```python
from build123d import *

# Parameters (mm, degrees)
DODANIE_WYCI_GNI_CIE1_DEPTH                 = 880
DODANIE_WYCI_GNI_CIE1_DEPTH_BACK            = 880
SZKIC1_R                                    = 12
WYTNIJ_WYCI_GNI_CIE1_REACH                  = 882.164
WYTNIJ_WYCI_GNI_CIE1_END_RADIUS             = 12
SZKIC2_R                                    = 4
WYTNIJ_WYCI_GNI_CIE1_DIRECTION_2_REACH      = 882.164
WYTNIJ_WYCI_GNI_CIE1_DIRECTION_2_END_RADIUS = 12
SFAZOWANIE1_SIZE                            = 1


with BuildPart() as part:
    # Szkic1 → Dodanie-wyciągnięcie1 (new, two sides: drawn at the far end of the back side and taken through both)
    with BuildSketch(Plane.XY.offset(-DODANIE_WYCI_GNI_CIE1_DEPTH_BACK)):
        Circle(SZKIC1_R)
    extrude(amount=DODANIE_WYCI_GNI_CIE1_DEPTH + DODANIE_WYCI_GNI_CIE1_DEPTH_BACK)

    # Wytnij-wyciągnięcie1: up to this cylinder (the profile starts inside it)
    wytnij_wyci_gni_cie1_end = Plane(origin=(0, 0, 0), z_dir=(0, 0, 1)) * Cylinder(WYTNIJ_WYCI_GNI_CIE1_END_RADIUS, 3529.328, mode=Mode.PRIVATE)
    # Szkic2 → Wytnij-wyciągnięcie1 (cut, up to the surface)
    with BuildSketch(Plane(origin=(0, 0, 0), x_dir=(1, 0, 0), z_dir=(0, 1, 0)), mode=Mode.PRIVATE) as wytnij_wyci_gni_cie1_sk1:
        with Locations(Location((0, 870, 0), (0, 0, 90))):
            Circle(SZKIC2_R)
    wytnij_wyci_gni_cie1_tool1 = extrude(wytnij_wyci_gni_cie1_sk1.sketch, amount=-WYTNIJ_WYCI_GNI_CIE1_REACH, mode=Mode.PRIVATE) & wytnij_wyci_gni_cie1_end
    add(wytnij_wyci_gni_cie1_tool1.solids().sort_by_distance((0, 0, -870))[0], mode=Mode.SUBTRACT)
    # Szkic2 → Wytnij-wyciągnięcie1 (cut, up to the surface)
    with BuildSketch(Plane(origin=(0, 0, 0), x_dir=(1, 0, 0), z_dir=(0, 1, 0)), mode=Mode.PRIVATE) as wytnij_wyci_gni_cie1_sk2:
        with Locations(Location((0, -870, 0), (0, 0, 90))):
            Circle(SZKIC2_R)
    wytnij_wyci_gni_cie1_tool2 = extrude(wytnij_wyci_gni_cie1_sk2.sketch, amount=-WYTNIJ_WYCI_GNI_CIE1_REACH, mode=Mode.PRIVATE) & wytnij_wyci_gni_cie1_end
    add(wytnij_wyci_gni_cie1_tool2.solids().sort_by_distance((0, 0, 870))[0], mode=Mode.SUBTRACT)

    # Wytnij-wyciągnięcie1 direction 2: up to this cylinder (the profile starts inside it)
    wytnij_wyci_gni_cie1_direction_2_end = Plane(origin=(0, 0, 0), z_dir=(0, 0, 1)) * Cylinder(WYTNIJ_WYCI_GNI_CIE1_DIRECTION_2_END_RADIUS, 3529.328, mode=Mode.PRIVATE)
    # Szkic2 → Wytnij-wyciągnięcie1 direction 2 (cut, up to the surface)
    with BuildSketch(Plane(origin=(0, 0, 0), x_dir=(1, 0, 0), z_dir=(0, 1, 0)), mode=Mode.PRIVATE) as wytnij_wyci_gni_cie1_direction_2_sk1:
        with Locations(Location((0, 870, 0), (0, 0, 90))):
            Circle(SZKIC2_R)
    wytnij_wyci_gni_cie1_direction_2_tool1 = extrude(wytnij_wyci_gni_cie1_direction_2_sk1.sketch, amount=WYTNIJ_WYCI_GNI_CIE1_DIRECTION_2_REACH, mode=Mode.PRIVATE) & wytnij_wyci_gni_cie1_direction_2_end
    add(wytnij_wyci_gni_cie1_direction_2_tool1.solids().sort_by_distance((0, 0, -870))[0], mode=Mode.SUBTRACT)
    # Szkic2 → Wytnij-wyciągnięcie1 direction 2 (cut, up to the surface)
    with BuildSketch(Plane(origin=(0, 0, 0), x_dir=(1, 0, 0), z_dir=(0, 1, 0)), mode=Mode.PRIVATE) as wytnij_wyci_gni_cie1_direction_2_sk2:
        with Locations(Location((0, -870, 0), (0, 0, 90))):
            Circle(SZKIC2_R)
    wytnij_wyci_gni_cie1_direction_2_tool2 = extrude(wytnij_wyci_gni_cie1_direction_2_sk2.sketch, amount=WYTNIJ_WYCI_GNI_CIE1_DIRECTION_2_REACH, mode=Mode.PRIVATE) & wytnij_wyci_gni_cie1_direction_2_end
    add(wytnij_wyci_gni_cie1_direction_2_tool2.solids().sort_by_distance((0, 0, 870))[0], mode=Mode.SUBTRACT)

    # Sfazowanie1
    sfazowanie1_edges = [part.edges().sort_by_distance(p)[0] for p in [
        (-12, 0, -880),
        (-12, 0, 880),
    ]]
    chamfer(sfazowanie1_edges, length=SFAZOWANIE1_SIZE)


solid = part.part
```
Work out the finished part from the listing and answer in its coordinate system (mm). Coordinates: 2 decimals unless noted, no trailing zeros. Write each loop counter-clockwise with the first axis right and the second up, starting at its lowest first coordinate (ties: lowest second). Pieces come first, ordered by that corner, then holes.
Q1. Find the intervals of material crossed by line 1 (Z direction, x = 1.5, y = -1); line 2 (Z direction, x = -3.25, y = -8.5); line 3 (X direction, y = -4.75, z = -7), in increasing order.
Q2. A cutting plane is placed at A-A, the plane z = -306.5. Give the vertices of the cut face in (x, y), then the cut area to 3 significant figures.
Q3. Each of these flat-tipped pins is pushed along its axis until it touches: pin 1 Ø8 at (y, z) = (9, 488.5) entering from +X; pin 2 Ø10 at (y, z) = (7, -92) entering from -X; pin 3 Ø12 at (x, z) = (8, -203.5) entering from +Y; pin 4 Ø5 at (x, z) = (0, -870) entering from +Y. Where does it stop, or does it pass through?
Q4. A cutting plane is placed at B-B, the plane y = -7.25. State how many separate pieces and enclosed holes the cut face has, then the cut area to 3 significant figures.
Findings below:
1. line 1: z = -880 to -873.71, -866.29 to 866.29, 873.71 to 880
1. line 2: z = -880 to -872.33, -867.67 to 867.67, 872.33 to 880
1. line 3: x = -11.02 to 11.02
2. outline: circle Ø24 at (0, 0)
2. area: 452 mm2
3. pin 1: stops at x = 10.91
3. pin 2: stops at x = -11.83
3. pin 3: stops at y = 11.83
3. pin 4: passes through
4. separate pieces: 1
4. enclosed holes: 2
4. area: 33,600 mm2
